The listing builds one solid part. Answer for the finished solid, in the listing's coordinates (mm). Coordinates: 2 decimals unless noted, no trailing zeros. Loops run counter-clockwise (first coordinate to the right, second up) from the corner with the lowest first, then second, coordinate; pieces in that order, holes last. Notation, with made-up numbers: M 85,60.5 L 98,60.5 A24 cw 98,88.5 Z; hole C 22.25,67.25 d4. An arc over 180 degrees is marked long. Answer as a JSON object with one key per item and string values. Group by question number.
1. Given pin 1 (4 mm diameter, centred on y = 16.5, z = 483.5, fed in from +X); pin 2 (4 mm diameter, centred on y = 21.5, z = 443.5, fed in from -X); pin 3 (6 mm diameter, centred on x = 229, z = 676, fed in from -Y), each flat-ended and moving along its own axis, determine where each tip first touches the part or whether it passes through.
2. A cutting plane is placed at B-B on z = 163. Give the vertices of the cut face in (x, y).
3. A cutting plane is placed at A-A on z = 441. Give the vertices of the cut face in (x, y), and give its area (3 significant figures).
4. Straight lines are drawn through the part: L1, parallel to X at y = 16.5, z = 357; L2, parallel to Z at x = 229, y = 21.5; L3, parallel to Y at x = 232, z = 656.5. For each, find the intervals that lie inside material, in ascending order.
from build123d import *

# Parameters (mm, degrees)
F0_R     = 7.1577178439
F0_R_2   = 6
F0_R_3   = 5
F0_R_4   = 4
F1_DEPTH = 200
F2_DEPTH = 400
F3_DEPTH = 600
F4_DEPTH = 800


# Not quite as in the source:
# - a fillet or chamfer that OpenCascade refuses, or shapes differently, is made with other operations: its cross-section is extruded or revolved along the edge and cut away or added


with BuildPart() as f1:
    # F0 (on Top) → F1 (new body)
    with BuildSketch(Plane.XY):
        with Locations((231.38127774, 15.8246317059)):
            Circle(F0_R)
        with Locations((231.38127774, 15.8246317059)):
            Circle(F0_R_2, mode=Mode.SUBTRACT)
        with Locations((231.38127774, 15.8246317059)):
            Circle(F0_R_2)
        with Locations((231.38127774, 15.8246317059)):
            Circle(F0_R_3, mode=Mode.SUBTRACT)
        with Locations((231.38127774, 15.8246317059)):
            Circle(F0_R_3)
        with Locations((231.38127774, 15.8246317059)):
            Circle(F0_R_4, mode=Mode.SUBTRACT)
        with Locations((231.38127774, 15.8246317059)):
            Circle(F0_R_4)
    extrude(amount=F1_DEPTH)

    # F0 (on Top) → F2 (join)
    with BuildSketch(Plane.XY):
        with Locations((231.38127774, 15.8246317059)):
            Circle(F0_R_2)
        with Locations((231.38127774, 15.8246317059)):
            Circle(F0_R_3, mode=Mode.SUBTRACT)
        with Locations((231.38127774, 15.8246317059)):
            Circle(F0_R_3)
        with Locations((231.38127774, 15.8246317059)):
            Circle(F0_R_4, mode=Mode.SUBTRACT)
        with Locations((231.38127774, 15.8246317059)):
            Circle(F0_R_4)
    extrude(amount=F2_DEPTH)

    # F0 (on Top) → F3 (join)
    with BuildSketch(Plane.XY):
        with Locations((231.38127774, 15.8246317059)):
            Circle(F0_R_3)
        with Locations((231.38127774, 15.8246317059)):
            Circle(F0_R_4, mode=Mode.SUBTRACT)
        with Locations((231.38127774, 15.8246317059)):
            Circle(F0_R_4)
    extrude(amount=F3_DEPTH)

    # F0 (on Top) → F4 (join)
    with BuildSketch(Plane.XY):
        with Locations((231.38127774, 15.8246317059)):
            Circle(F0_R_4)
    extrude(amount=F4_DEPTH)

    # F5: fillet of radius 2 on 4 edges, made by hand

    # F5_s1 → F5_t2 (revolve, cut)
    with BuildSketch(Plane.XZ.offset(-15.8246317059)):
        with BuildLine():
            ThreePointArc((238.5393955839, 198.1853934994), (238.2252538415, 199.261841349), (237.3814463082, 200.0003627462))
            Line((237.3814463082, 200.0003627462), (237.4657879491, 200.1818596708))
            ThreePointArc((237.4657879491, 200.1818596708), (237.9602209461, 200.2001365685), (238.5389955839, 200.2001365685))
            Line((238.5389955839, 200.2001365685), (238.7391321525, 200))
            ThreePointArc((238.7391321525, 200), (238.7391321525, 199.0926967497), (238.7395321525, 198.1853934994))
            Line((238.7395321525, 198.1853934994), (238.5393955839, 198.1853934994))
        make_face()
    revolve(axis=Axis((231.38127774, 15.8246317059, 200), (0, 0, 1)), mode=Mode.SUBTRACT)

    # F5_s3 → F5_t4 (revolve, cut)
    with BuildSketch(Plane.XZ.offset(-15.8246317059)):
        with BuildLine():
            ThreePointArc((237.38167774, 398.2673917434), (237.1136849874, 399.2678330874), (236.3814778365, 400.0003463544))
            Line((236.3814778365, 400.0003463544), (236.4815944147, 400.1736418155))
            ThreePointArc((236.4815944147, 400.1736418155), (236.8813777883, 400.2001365685), (237.38127774, 400.2001365685))
            Line((237.38127774, 400.2001365685), (237.5814143085, 400))
            ThreePointArc((237.5814143085, 400), (237.5814143085, 399.1336958717), (237.5818143085, 398.2673917434))
            Line((237.5818143085, 398.2673917434), (237.38167774, 398.2673917434))
        make_face()
    revolve(axis=Axis((231.38127774, 15.8246317059, 400), (0, 0, 1)), mode=Mode.SUBTRACT)

    # F5_s5 → F5_t6 (revolve, cut)
    with BuildSketch(Plane.XZ.offset(-15.8246317059)):
        with BuildLine():
            ThreePointArc((236.38167774, 598.2673917434), (236.1136849874, 599.2678330874), (235.3814778365, 600.0003463544))
            Line((235.3814778365, 600.0003463544), (235.4815944147, 600.1736418155))
            ThreePointArc((235.4815944147, 600.1736418155), (235.8813777883, 600.2001365685), (236.38127774, 600.2001365685))
            Line((236.38127774, 600.2001365685), (236.5814143085, 600))
            ThreePointArc((236.5814143085, 600), (236.5814143085, 599.1336958717), (236.5818143085, 598.2673917434))
            Line((236.5818143085, 598.2673917434), (236.38167774, 598.2673917434))
        make_face()
    revolve(axis=Axis((231.38127774, 15.8246317059, 600), (0, 0, 1)), mode=Mode.SUBTRACT)

    # F5_s7 → F5_t8 (revolve, cut)
    with BuildSketch(Plane.XZ.offset(-15.8246317059)):
        with BuildLine():
            ThreePointArc((235.38167774, 797.9990343146), (234.7954913024, 799.4142135624), (233.3803120546, 800.0004))
            Line((233.3803120546, 800.0004), (233.3803120546, 800.2005365685))
            ThreePointArc((233.3803120546, 800.2005365685), (234.3807948973, 800.2001365685), (235.38127774, 800.2001365685))
            Line((235.38127774, 800.2001365685), (235.5814143085, 800))
            ThreePointArc((235.5814143085, 800), (235.5814143085, 798.9995171573), (235.5818143085, 797.9990343146))
            Line((235.5818143085, 797.9990343146), (235.38167774, 797.9990343146))
        make_face()
    revolve(axis=Axis((231.38127774, 15.8246317059, 800), (0, 0, 1)), mode=Mode.SUBTRACT)


solid = f1.part
From the geometry:
{
 "1": {"pin 1": "stops at x = 236.38", "pin 2": "stops at x = 227.99", "pin 3": "stops at y = 11.82"},
 "2": {"outline": "C 231.38,15.82 d14.32"},
 "3": {"outline": "C 231.38,15.82 d10", "area": "78.5 mm²"},
 "4": {"L1": "x = 225.42 to 237.34", "L2": "z = 0 to 199.92", "L3": "y = 11.87 to 19.78"}
}
